Could you check a few things on this model? Use its own coordinates, in mm. A direction names the side the tool comes from. Coordinates: 2 decimals unless noted, no trailing zeros. Loops run counter-clockwise (first coordinate to the right, second up) from the corner with the lowest first, then second, coordinate; pieces in that order, holes last. Notation, with made-up numbers: (2, 74.5) -> (21, 74.5) arc R10 ccw to (21, 82.5) -> close; hole circle Ø11 at (25.25, 32). An arc over 180 degrees is marked (long way). One line per question, with ' | ' between items.
Autodesk Inventor part; units mm, degrees
ref_plane "YZ Plane" through (0, 0, 0) normal (1, 0, 0) x (0, 1, 0)
ref_plane "XZ Plane" through (0, 0, 0) normal (0, 1, 0) x (-1, 0, 0)
ref_plane "XY Plane" through (0, 0, 0) normal (0, 0, 1) x (1, 0, 0)
sketch "Sketch1" plane through (0, 0, 0) normal (0, 1, 0) x (-1, 0, 0)
  line L0 (-10.3707, 15.395) -> (-8.7381, 17.0275)
  arc A0 (-7.8549, 16.6) -> (-8.7381, 17.0275) centre (-8.4, 16.6) ccw
  line L1 (-7.8549, 16.6) -> (-7.8549, 15.135)
  line L2 (-7.8549, 15.135) -> (-6.3429, 15.135)
  line L3 (-6.3429, 15.135) -> (-4.3451, 17.1329)
  line L4 (-4.3451, 17.1329) -> (-4.3451, 22.8671)
  line L5 (-4.3451, 22.8671) -> (-6.3429, 24.865)
  line L6 (-6.3429, 24.865) -> (-7.8549, 24.865)
  line L7 (-7.8549, 24.865) -> (-7.8549, 23.8568)
  arc A1 (-9.0499, 23.3618) -> (-7.8549, 23.8568) centre (-8.5549, 23.8568) ccw
  line L8 (-9.0499, 23.3618) -> (-10.3707, 24.6827)
  line L9 (-10.3707, 15.395) -> (-10.3707, 10.0707)
  line L10 (-10.3707, 10.0707) -> (-12.399, 10.0707)
  line L11 (-10.3707, 10.0707) -> (-18.3707, 10.0707)
  line L12 (-18.3707, 10.0707) -> (-18.3707, 50.0707)
  line L13 (-18.3707, 50.0707) -> (-14.3707, 50.0707)
  line L14 (-10.3707, 15.395) -> (-10.3707, 10.0707)
  line L15 (-14.3707, 50.0707) -> (-14.3707, 28.6827)
  line L16 (-14.3707, 28.6827) -> (-10.3707, 24.6827)
  line L17 (-10.3707, 24.6827) -> (-10.3707, 24.865)
  line L18 (-10.3707, 50.0707) -> (-10.3707, 28.8927)
  line L19 (-10.3707, 24.865) -> (-10.3707, 24.6827)
  point P0 (0, 0)
  point P1 (-9.0499, 23.3618)
  dimension "d5" = 40
extrude "Extrusion1" add sketch "Sketch1" along normal blind 25
sketch "Sketch3" plane through (10.3707, 0, 10.0707) normal (0, 0, -1) x (-1, 0, 0)
  point P0 (10.3707, 0)
fillet "Fillet1" radius 3 1 edges at (18.3707, 12.5, 10.0707)
fillet "Fillet2" radius 3 1 edges at (18.3707, 12.5, 50.0707)
properties part number "LED Mount"
1) I need wall thicknesses on line 1 along Z through (x, y) = (8.5, 3.75); line 2 along X through (y, z) = (17.25, 37); line 3 along Z through (x, y) = (7, 11) (3 decimals). Which ranges of each line are inside material? Lowest first, please. Write a range as from..to.
Data:
line 1: 17.14..23.16 | line 2: 14.37..18.37 | line 3: 15.135..24.865
2) We'd pull the mould along X, two halves only. Please class faces 4 (the face through (13, 12, 10.071)), 5 (the face through (4.345, 12, 20)), 6 (the face through (8.17, 12.325, 17.094)): pulls with the +X half, pulls with the -X half, needs draft (parallel to the pull), parting line crosses it, or undercut.
Data:
face 4: needs draft | face 5: pulls with the -X half | face 6: undercut
3) On a 3-axis mill with a long thin cutter (end or side, diameter ignored), from which of +Z, -Z, +X, -X, +Y, -Y can I reach the whole of each face in a straight line? I mean faces 1 (the face through (9.566, 12.325, 16.2)), 2 (the face through (7.855, 12.3, 24.4)), 3 (the face through (7, 12, 24.865)). Say none if no direction works.
Data:
face 1: -Z, +Y, -Y | face 2: +Z, +Y, -Y | face 3: +Z, -X, +Y, -Y
4) If we section it at A-A on y = 7.75: Please give me the cut outline in (x, z) (1 decimal).
Data:
outline: (4.3, 17.1) -> (6.3, 15.1) -> (7.9, 15.1) -> (7.9, 16.6) arc R0.5 cw to (8.7, 17) -> (10.4, 15.4) -> (10.4, 10.1) -> (15.4, 10.1) arc R3 ccw to (18.4, 13.1) -> (18.4, 47.1) arc R3 ccw to (15.4, 50.1) -> (14.4, 50.1) -> (14.4, 28.7) -> (10.4, 24.7) -> (9, 23.4) arc R0.7 cw to (7.9, 23.9) -> (7.9, 24.9) -> (6.3, 24.9) -> (4.3, 22.9) -> close
5) If we section it at C-C on x = 13.75: Please give me the cut outline in (y, z).
Data:
outline: (0, 10.07) -> (25, 10.07) -> (25, 28.06) -> (0, 28.06) -> close
6) I'm going to push flat-ended pins straight in: pin 1 Ø1.7 at (x, y) = (7, 9.5) entering from -Z (3 decimals); pin 2 Ø1.6 at (y, z) = (15, 12.5) entering from -X; pin 3 Ø1.2 at (x, y) = (7, 10) entering from +Z (3 decimals). Where does each tip first touch, or does it pass through?
Data:
pin 1: z = 15.135 | pin 2: x = 10.37 | pin 3: z = 24.865
7) If we section it at B-B on z = 36.5: Please give me the cut outline in (x, y), and give its area (3 significant figures).
Data:
outline: (14.37, 0) -> (18.37, 0) -> (18.37, 25) -> (14.37, 25) -> close | area: 100 mm²
